The figure shows three views and two pictorial views of one solid part (mm, origin at its lowest corner). Answer the questions. A direction names the side the tool comes from. Coordinates: 2 decimals unless noted, no trailing zeros. Order: outer loops, then holes, each group sorted by start corner. A loop starts at its lowest first (then second) coordinate and runs counter-clockwise, first axis right, second up. Notation, with made-up numbers: (69.25, -8) - (82.25, -8) arc R7 ccw to (82.25, -3) - close; hole circle Ø1 at (10, 41). An arc over 180 degrees is marked (long way). Answer as a JSON object with one key per item and string values. Group by question number.
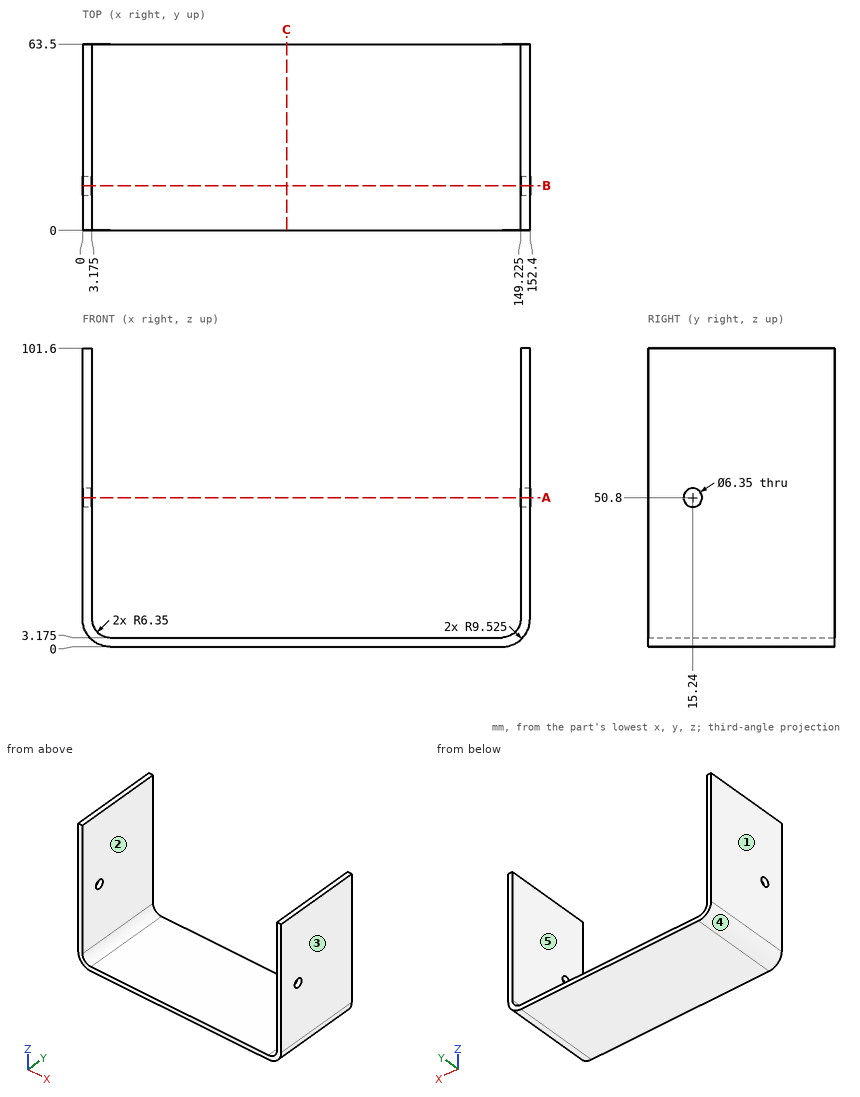
1. Given pin 1 (5 mm diameter, centred on x = 38, y = 36.5, fed in from +Z) (3 decimals), flat-ended and moving along its own axis, determine where the tip first touches the part or whether it passes through.
2. A cutting plane is placed at A-A on z = 50.8. Write down the section's boundary in (x, y) (3 decimals).
3. A cutting plane is placed at C-C on x = 69.5. Write down the section's boundary in (y, z) (3 decimals), and give its area (3 significant figures).
4. A cutting plane is placed at B-B on y = 15.24. Write down the section's boundary in (x, z) (3 decimals), and give its area (3 significant figures).
5. For a pull along X with two mould halves and no side action, classify the marked faces 3, 4 and 5 as pulls with the +X half, pulls with the -X half, needs draft (parallel to the pull), parting line crosses it, or undercut.
6. For the marked faces 1 and 2, determine the directions among +Z, -Z, +X, -X, +Y, -Y from which every point of the face is accessible in a straight line to the end or side of a thin tool.
7. Straight lines are drawn through the part: L1, parallel to Y at x = 150.8, z = 50.8 (3 decimals); L2, parallel to X at y = 44.5, z = 40 (3 decimals); L3, parallel to Z at x = 9, y = 22.5. For each, find the intervals that lie inside material, in ascending order.
Derived:
{
 "1": {"pin 1": "stops at z = 3.175"},
 "2": {"outline": "(0, 0) - (3.175, 0) - (3.175, 12.065) - (0, 12.065) - close; (0, 18.415) - (3.175, 18.415) - (3.175, 63.5) - (0, 63.5) - close; (149.225, 0) - (152.4, 0) - (152.4, 12.065) - (149.225, 12.065) - close; (149.225, 18.415) - (152.4, 18.415) - (152.4, 63.5) - (149.225, 63.5) - close"},
 "3": {"outline": "(0, 0) - (63.5, 0) - (63.5, 3.175) - (0, 3.175) - close", "area": "202 mm2"},
 "4": {"outline": "(0, 9.525) arc R9.525 ccw to (9.525, 0) - (142.875, 0) arc R9.525 ccw to (152.4, 9.525) - (152.4, 47.625) - (149.225, 47.625) - (149.225, 9.525) arc R6.35 cw to (142.875, 3.175) - (9.525, 3.175) arc R6.35 cw to (3.175, 9.525) - (3.175, 47.625) - (0, 47.625) - close; (0, 53.975) - (3.175, 53.975) - (3.175, 101.6) - (0, 101.6) - close; (149.225, 53.975) - (152.4, 53.975) - (152.4, 101.6) - (149.225, 101.6) - close", "area": "1,050 mm2"},
 "5": {"face 3": "pulls with the +X half", "face 4": "pulls with the -X half", "face 5": "undercut"},
 "6": {"face 1": "+Z, -Z, -X, +Y, -Y", "face 2": "+Z, +Y, -Y"},
 "7": {"L1": "y = 0 to 12.065, 18.415 to 63.5", "L2": "x = 0 to 3.175, 149.225 to 152.4", "L3": "z = 0.01 to 3.2"}
}
